Part model, mm, in its own coordinate system. A direction names the side the tool comes from. Give positions to 0.01 mm unless a question says otherwise; leave off trailing zeros. Order: outer loops, then holes, each group sorted by start corner. A loop starts at its lowest first (then second) coordinate and runs counter-clockwise, first axis right, second up. Notation, with made-up numbers: M 3.25,58 L 36.25,58 A17 ccw 36.25,90 Z; hole C 49.5,85 d3. An arc over 180 degrees is marked long. Return JSON: item names as keys, results as strings.
from build123d import *

# Parameters (mm, degrees)
SKETCH1_R           = 13.35
SKETCH1_R_2         = 11.35
EXTRUDE_THIN1_DEPTH = 13
BOSS_EXTRUDE1_DEPTH = 5
SKETCH3_R           = 10.65
SKETCH3_R_2         = 8.65
EXTRUDE_THIN2_DEPTH = 20


with BuildPart() as part:
    # Sketch1 → Extrude-Thin1 (new, symmetric)
    with BuildSketch(Plane.XY):
        Circle(SKETCH1_R)
        Circle(SKETCH1_R_2, mode=Mode.SUBTRACT)
    extrude(amount=EXTRUDE_THIN1_DEPTH, both=True)

    # Sketch2 → Boss-Extrude1 (add, symmetric)
    with BuildSketch(Plane.XY.offset(13)):
        Polygon((15.942171509, 8.387348964), (0.707428481, 18), (-15.234743028, 9.612651036), (-15.942171509, -8.387348964), (-0.707428481, -18), (15.234743028, -9.612651036), align=None)
    extrude(amount=BOSS_EXTRUDE1_DEPTH, both=True)

    # Sketch3 → Extrude-Thin2 (add)
    with BuildSketch(Plane.XY.offset(18)):
        Circle(SKETCH3_R)
        Circle(SKETCH3_R_2, mode=Mode.SUBTRACT)
    extrude(amount=EXTRUDE_THIN2_DEPTH)


solid = part.part
Q1. Probe line 1 along Y through (x, z) = (0, 2); line 2 along Y through (x, z) = (0, 31); line 3 along Z through (x, y) = (-11, 9). List the from-to ranges inside material, lowest first.
Established:
{"line 1": "y = -13.35 to -11.35, 11.35 to 13.35", "line 2": "y = -10.65 to -8.65, 8.65 to 10.65", "line 3": "z = 8 to 18"}
Q2. 3-axis set-ups, long thin cutter, end or side, ignore diameter. For faces 5 (the flat face through (0, 0, 18)), 6 (the cylindrical face through (12.734, 4.01, -2.353)), 7 (the flat face through (7.152, -13.865, 13.07)): which of +Z, -Z, +X, -X, +Y, -Y reach the whole face in a straight line?
Established:
{"face 5": "+Z", "face 6": "-Z", "face 7": "+Z, -Z, +X, -Y"}
Q3. Two-plate mould, pull along Y, no slides. Class faces 1 (the flat face through (-8.431, -13.126, 13.07)), 2 (the flat face through (0, 9, 38)), 3 (the cylindrical face through (10.485, -4.347, -2.647)), 4 (the flat face through (-7.152, 13.865, 13.07)): +Y half, -Y half, draft (parallel to the pull), parting line (faces both ways), or undercut.
Established:
{"face 1": "-Y half", "face 2": "draft", "face 3": "undercut", "face 4": "+Y half"}
Q4. Pin check, flat tips, straight feed: pin 1 (12 mm diameter, centred on x = -5.5, z = -0.5, fed in from -Y); pin 2 (7 mm diameter, centred on x = -3.5, y = 0, fed in from -Z); pin 3 (3 mm diameter, centred on x = 9.5, y = 9.5, fed in from +Z); pin 4 (5 mm diameter, centred on x = -4.5, y = -8, fed in from -Z). Stop position of each tip, or through.
Established:
{"pin 1": "stops at y = -13.35", "pin 2": "stops at z = 8", "pin 3": "stops at z = 18", "pin 4": "stops at z = -13"}
Q5. Band-saw the part on B-B (y = 3). Give the cut face in (x, z).
Established:
{"outline": "M -15.49,8 L -13.01,8 L -13.01,-13 L -10.95,-13 L -10.95,8 L 10.95,8 L 10.95,-13 L 13.01,-13 L 13.01,8 L 15.73,8 L 15.73,18 L 10.22,18 L 10.22,38 L 8.11,38 L 8.11,18 L -8.11,18 L -8.11,38 L -10.22,38 L -10.22,18 L -15.49,18 Z"}
Q6. Band-saw the part on D-D (z = -3.5). Give the cut face in (x, y).
Established:
{"outline": "C 0,0 d26.7; hole C 0,0 d22.7"}
Q7. Band-saw the part on C-C (x = 6.5). Give the cut face in (y, z).
Established:
{"outline": "M -14.21,8 L -11.66,8 L -11.66,-13 L -9.3,-13 L -9.3,8 L 9.3,8 L 9.3,-13 L 11.66,-13 L 11.66,8 L 14.35,8 L 14.35,18 L 8.44,18 L 8.44,38 L 5.71,38 L 5.71,18 L -5.71,18 L -5.71,38 L -8.44,38 L -8.44,18 L -14.21,18 Z"}
Q8. Band-saw the part on A-A (z = 33.5). Give the cut face in (x, y).
Established:
{"outline": "C 0,0 d21.3; hole C 0,0 d17.3"}
